The figure shows three views and two pictorial views of one solid part (mm, origin at its lowest corner). Answer the questions. Coordinates: 2 decimals unless noted, no trailing zeros. Write each loop counter-clockwise with the first axis right and the second up, starting at its lowest first coordinate (ties: lowest second). Pieces come first, ordered by that corner, then holes.
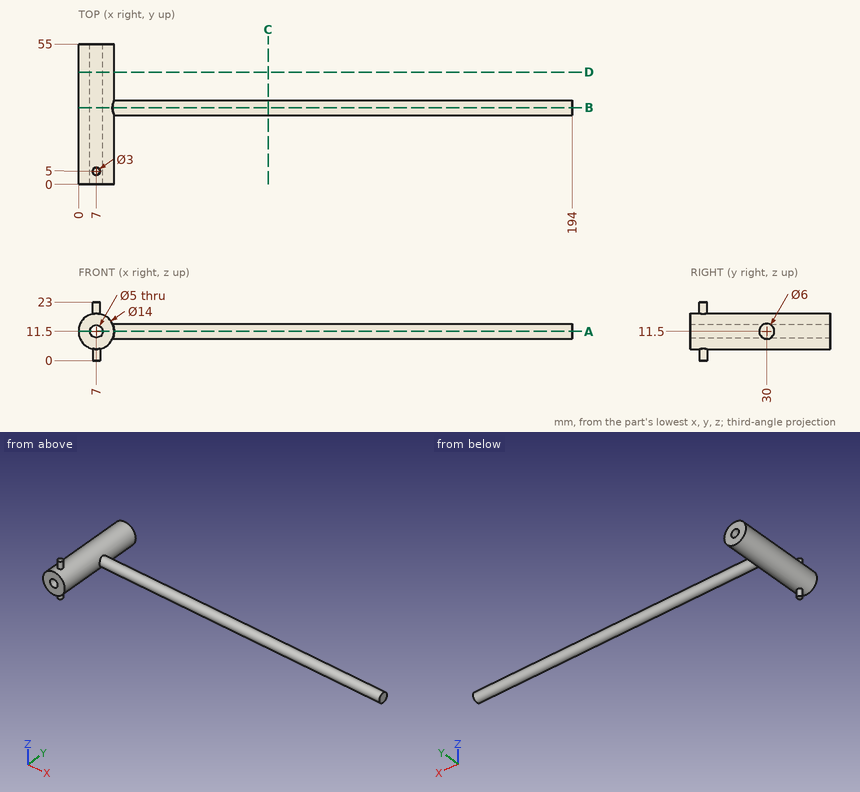
1. Find the intervals of material crossed by L1, parallel to X at y = 13, z = 11.5; L2, parallel to X at y = 30, z = 11.5; L3, parallel to Y at x = 95, z = 14, in increasing order.
Results found:
L1: x = 0 to 4.5, 9.5 to 14
L2: x = 0 to 4.5, 9.5 to 194
L3: y = 28.34 to 31.66
2. Flat-ended cylindrical pins translate along their axes: P1, Ø3, axis at x = 108, y = 35, coming from the -Z side; P2, Ø4, axis at y = 45.5, z = 11, coming from the +X side; P3, Ø6, axis at x = 89, y = 26, coming from the +Z side; P4, Ø8, axis at x = 104, z = 7.5, coming from the +Y side. Find the tip coordinate at first contact, or state that the pin passes through.
Results found:
P1: passes through
P2: stops at x = 14
P3: stops at z = 14.33
P4: stops at y = 33
3. Section A-A on z = 11.5 is taken. Give the vertices of the cut face in (x, y).
Results found:
outline: (0, 0) - (4.5, 0) - (4.5, 55) - (0, 55) - close; (9.5, 0) - (14, 0) - (14, 27) - (194, 27) - (194, 33) - (14, 33) - (14, 55) - (9.5, 55) - close
4. Section B-B on y = 30 is taken. Give the vertices of the cut face in (x, z).
Results found:
outline: (13.32, 8.5) - (194, 8.5) - (194, 14.5) - (13.32, 14.5) arc R7 ccw (long way) to start; hole circle Ø5 at (7, 11.5)
5. Section C-C on x = 74.5 is taken. Give the vertices of the cut face in (y, z), then the cut area to 3 significant figures.
Results found:
outline: circle Ø6 at (30, 11.5)
area: 28.3 mm2
6. Section D-D on y = 44 is taken. Give the vertices of the cut face in (x, z).
Results found:
outline: circle Ø14 at (7, 11.5); hole circle Ø5 at (7, 11.5)
